Verification items for the finished model (mm, model axes). Face numbers are marked on the shaded views. A direction names the side the tool comes from. Coordinates: 2 decimals unless noted, no trailing zeros. Loops run counter-clockwise (first coordinate to the right, second up) from the corner with the lowest first, then second, coordinate; pieces in that order, holes last. Notation, with made-up numbers: (35, -23.75) -> (66, -23.75) arc R21 ccw to (66, 1.25) -> close; hole circle Ø11 at (82.5, 4). An arc over 180 degrees is marked (long way). Answer as a JSON object with one key per item and string values. Group by question number.
Q1. Cross-section at D-D on y = 7. Record the boundary of the cut face in (x, z), and give its area (3 significant figures).
Q2. Gauge pin test, flat ends, axial feed: pin 1 Ø1.8 at (x, z) = (26, 0) entering from +Y; pin 2 Ø0.9 at (y, z) = (4, 1.5) entering from +X. Record the tip position at first contact, or that the pin passes through.
Q3. Scan lines: L1, parallel to Z at x = 30.5, y = 3.5; L2, parallel to Y at x = 57.5, z = -0.5; L3, parallel to X at y = 3.25, z = 1. Record each from-to range of solid material in increasing order.
Q4. Cross-section at B-B on x = 30. Record the boundary of the cut face in (y, z), and give its area (3 significant figures).
Q5. Release check for a two-part mould opening along X. For the marked faces 1, 2, 3 and 4 record: released by +X, released by -X, zero draft, split by the parting line, or undercut.
Q6. Cross-section at C-C on z = 0. Record the boundary of the cut face in (x, y).
Q7. Cross-section at A-A on y = 2.75. Record the boundary of the cut face in (x, z), and give its area (3 significant figures).
Q8. Set-up check for the marked faces 5, 6 and 7: record each of +Z, -Z, +X, -X, +Y, -Y from which the full face is reachable in a straight line by a thin tool's end or side.
```python
from build123d import *

# Parameters (mm, degrees)
BOSS_EXTRUDE2_DEPTH     = 2
SKETCH3_W               = 30
SKETCH3_H               = 8
BOSS_EXTRUDE3_DEPTH     = 3
SKETCH4_R               = 1.5
BOSS_EXTRUDE4_DEPTH     = 7
SKETCH12_R              = 1.5
BOSS_EXTRUDE6_DEPTH     = 4
CUT_EXTRUDE1_DEPTH      = 71.042844031
CUT_EXTRUDE2_DEPTH      = 2
CUT_EXTRUDE2_DEPTH_BACK = 2


with BuildPart() as part:
    # Sketch1 → Boss-Extrude2 (new body)
    with BuildSketch(Plane(origin=(0, 0, 0), x_dir=(1, 0, 0), z_dir=(0, 1, 0))):
        with BuildLine():
            Line((25, -4), (65, -4))
            ThreePointArc((65, -4), (69, 0), (65, 4))
            Line((65, 4), (25, 4))
            Line((25, 4), (25, -4))
        make_face()
    extrude(amount=BOSS_EXTRUDE2_DEPTH)

    # Sketch3 → Boss-Extrude3 (add)
    with BuildSketch(Plane(origin=(0, 2, 0), x_dir=(1, 0, 0), z_dir=(0, 1, 0))):
        with Locations((40, 0)):
            Rectangle(SKETCH3_W, SKETCH3_H)
    extrude(amount=BOSS_EXTRUDE3_DEPTH)

    # Sketch4 → Boss-Extrude4 (add)
    with BuildSketch(Plane(origin=(0, 2, 0), x_dir=(1, 0, 0), z_dir=(0, 1, 0))):
        with Locations(Location((65, 0, 0), (0, 0, 270))):
            Circle(SKETCH4_R)
    extrude(amount=BOSS_EXTRUDE4_DEPTH)

    # Sketch12 → Boss-Extrude6 (add)
    with BuildSketch(Plane(origin=(0, 5, 0), x_dir=(1, 0, 0), z_dir=(0, 1, 0))):
        with Locations(Location((47, 0, 0), (0, 0, 270))):
            Circle(SKETCH12_R)
    extrude(amount=BOSS_EXTRUDE6_DEPTH)

    # Sketch13 → Cut-Extrude1 (cut, through all)
    with BuildSketch(Plane.XY.offset(4)):
        with BuildLine():
            Line((31.5, 5), (28.5, 5))
            ThreePointArc((28.5, 5), (30, 3.5), (31.5, 5))
        make_face()
    extrude(amount=-CUT_EXTRUDE1_DEPTH, mode=Mode.SUBTRACT)

    # Sketch14 → Cut-Extrude2 (cut, two sides: drawn at the far end of the back side and taken through both)
    with BuildSketch(Plane.XY.offset(-CUT_EXTRUDE2_DEPTH_BACK)):
        with BuildLine():
            Line((27, 5), (33, 5))
            ThreePointArc((33, 5), (30, 2), (27, 5))
        make_face()
    extrude(amount=CUT_EXTRUDE2_DEPTH + CUT_EXTRUDE2_DEPTH_BACK, mode=Mode.SUBTRACT)


solid = part.part
```
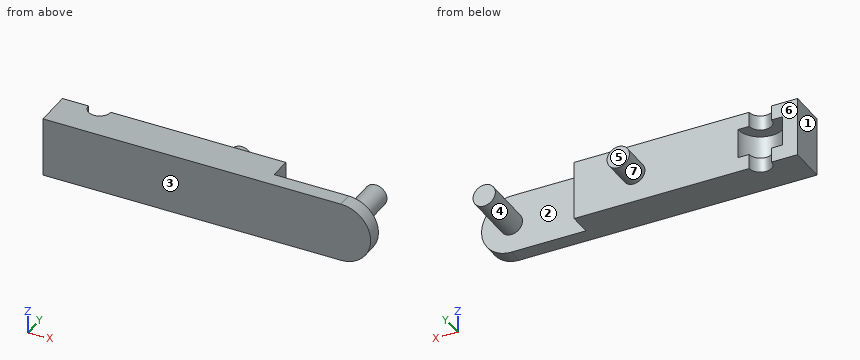
Computed values:
{
 "1": {"outline": "circle Ø3 at (47, 0); circle Ø3 at (65, 0)", "area": "14.1 mm²"},
 "2": {"pin 1": "stops at y = 5", "pin 2": "stops at x = 66.07"},
 "3": {"L1": "z = -4 to -2, 2 to 4", "L2": "y = 0 to 2", "L3": "x = 25 to 27.56, 32.44 to 55, 63.88 to 66.12"},
 "4": {"outline": "(0, -4) -> (3.5, -4) -> (3.5, -2) -> (2, -2) -> (2, 2) -> (3.5, 2) -> (3.5, 4) -> (0, 4) -> close", "area": "22.0 mm²"},
 "5": {"face 1": "released by -X", "face 2": "undercut", "face 3": "zero draft", "face 4": "undercut"},
 "6": {"outline": "(25, 0) -> (69, 0) -> (69, 2) -> (66.5, 2) -> (66.5, 9) -> (63.5, 9) -> (63.5, 2) -> (55, 2) -> (55, 5) -> (48.5, 5) -> (48.5, 9) -> (45.5, 9) -> (45.5, 5) -> (33, 5) arc R3 cw to (27, 5) -> (25, 5) -> close"},
 "7": {"outline": "(25, -4) -> (55, -4) -> (55, 4) -> (25, 4) -> close; circle Ø3 at (65, 0); hole (28.02, -2) -> (31.98, -2) -> (31.98, 2) -> (28.02, 2) -> close", "area": "231 mm²"},
 "8": {"face 5": "+Z, -Z, +X, -X, +Y", "face 6": "+Z, -Z, -X, +Y", "face 7": "+Y"}
}
